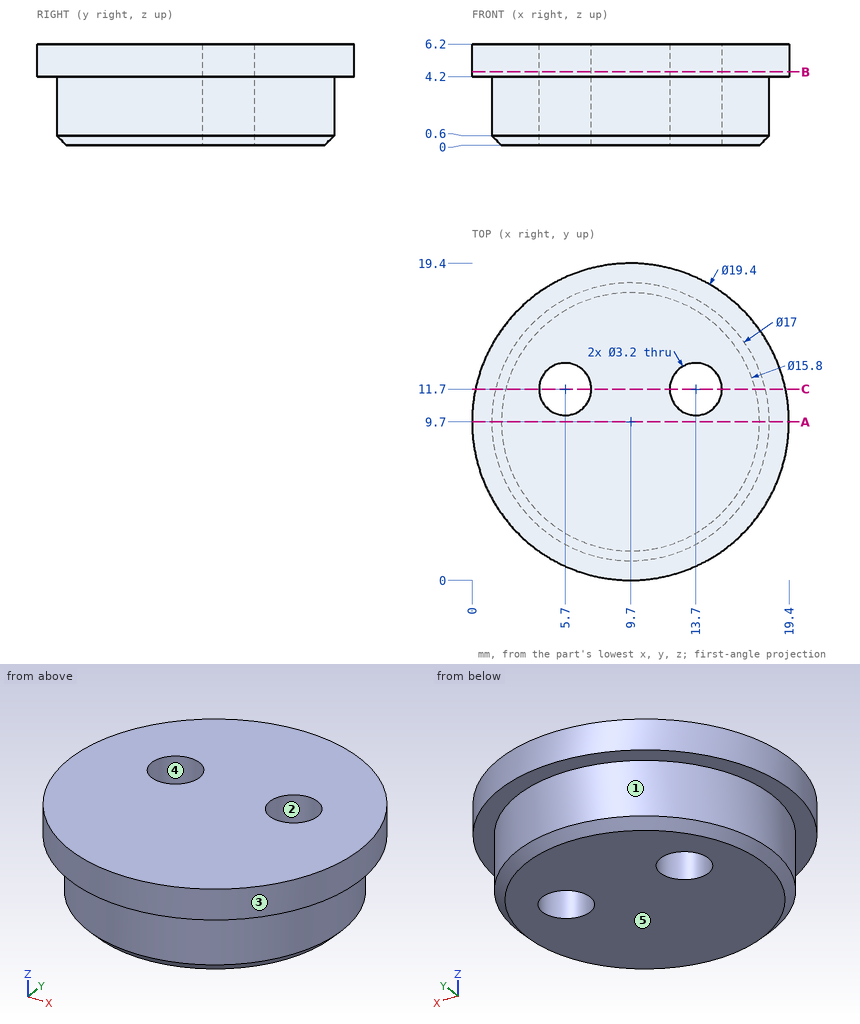
Geometry: see drawing. Coordinates: mm, zero at the bounding-box minimum. A direction names the side the tool comes from. Coordinates: 2 decimals unless noted, no trailing zeros. Loops run counter-clockwise (first coordinate to the right, second up) from the corner with the lowest first, then second, coordinate; pieces in that order, holes last. Notation, with made-up numbers: (15.5, 8.25) -> (49.5, 8.25) arc R26 ccw to (49.5, 36.25) -> close; hole circle Ø8 at (-32, -36.5). An arc over 180 degrees is marked (long way). Use a Markdown table: item, result.
1) Pull-direction query (Y, two-part tool) for the marked faces 3, 4 and 5; classes: released by +Y, released by -Y, zero draft, split by the parting line, or undercut.
Results found:
| item | result |
|---|---|
| face 3 | split by the parting line |
| face 4 | undercut |
| face 5 | zero draft |
2) Material intervals for line 1 along X through (y, z) = (13, 3); line 2 along Y through (x, z) = (5.7, 4.75); line 3 along Z through (x, y) = (9.25, 18.5), sorted ascending. Write a range as from..to.
Results found:
| item | result |
|---|---|
| line 1 | x = 1.87..4.77, 6.63..12.77, 14.63..17.53 |
| line 2 | y = 0.86..10.1, 13.3..18.54 |
| line 3 | z = 4.2..6.2 |
3) Cut plane B-B (z = 4.5). Return the cut outline in (x, y), then the cut area to 3 significant figures.
Results found:
| item | result |
|---|---|
| outline | circle Ø19.4 at (9.7, 9.7); hole circle Ø3.2 at (5.7, 11.7); hole circle Ø3.2 at (13.7, 11.7) |
| area | 280 mm2 |
4) Contact query for a flat-ended pin moving along its axis: pin 1 (2 mm diameter, centred on x = 5, z = 3, fed in from -Y). Output: stop coordinate, or through.
Results found:
| item | result |
|---|---|
| pin 1 | stops at y = 2.05 |
5) Cut plane A-A (y = 9.7). Return the cut outline in (x, z), then the cut area to 3 significant figures.
Results found:
| item | result |
|---|---|
| outline | (0, 4.2) -> (1.2, 4.2) -> (1.2, 0.6) -> (1.8, 0) -> (17.6, 0) -> (18.2, 0.6) -> (18.2, 4.2) -> (19.4, 4.2) -> (19.4, 6.2) -> (0, 6.2) -> close |
| area | 110 mm2 |
6) Cut plane C-C (y = 11.7). Give the number of separate pieces and of enclosed holes in the cut face, then the cut area to 3 significant figures.
Results found:
| item | result |
|---|---|
| separate pieces | 3 |
| enclosed holes | 0 |
| area | 67.3 mm2 |
7) Access query for the marked faces 1 and 2. Directions: +Z, -Z, +X, -X, +Y, -Y. A direction counts if a zero-diameter tool reaches every point of the face in a straight line with its end or side. Return the directions, or none.
Results found:
| item | result |
|---|---|
| face 1 | -Z |
| face 2 | +Z, -Z |
